Read the model definition and answer for the solid it produces. Units are mm, in the model's axes. Coordinates: 2 decimals unless noted, no trailing zeros. Loops run counter-clockwise (first coordinate to the right, second up) from the corner with the lowest first, then second, coordinate; pieces in that order, holes last. Notation, with made-up numbers: (61.25, -36) - (70.25, -36) arc R28 cw to (70.25, -15) - close; hole circle Ø8 at (-37.75, 28.25). An arc over 180 degrees is marked (long way). Use one line per item in the form item = value. Start each with the question number.
1) Each of these flat-tipped pins is pushed along its axis until it touches: P1, Ø3.5, axis at x = 137, y = 64, coming from the +Z side; P2, Ø1, axis at x = 16, z = 1.5, coming from the -Y side; P3, Ø1.5, axis at y = 72, z = 2, coming from the -X side. Where does it stop, or does it pass through?
2) A cutting plane is placed at A-A (y = 15). Give the vertices of the cut face in (x, z), and give its area (3 significant figures).
3) A cutting plane is placed at D-D (z = 2.1). State how many separate pieces and enclosed holes the cut face has, and give its area (3 significant figures).
4) The mould has two halves that part along X. Classify faces 1 (the face through (63, 37, 0)), 2 (the face through (106.05, 39.72, 1.52)), 3 (the face through (135.526, 65.352, 1.521)): released by +X, released by -X, zero draft, split by the parting line, or undercut.
5) Consider line 1 (X direction, y = 47.5, z = 1.45); line 2 (X direction, y = 66.5, z = 0.75); line 3 (Y direction, x = 88.5, z = 1.35). Determine where each line is inside the solid, lowest interval first.
6) A cutting plane is placed at C-C (y = 54). Give the vertices of the cut face in (x, z).
7) A cutting plane is placed at B-B (x = 137). Give the vertices of the cut face in (y, z).
from build123d import *

# Parameters (mm, degrees)
SKETCH1_R           = 5
BOSS_EXTRUDE1_DEPTH = 3
SKETCH2_R           = 2
SKETCH2_R_2         = 19
SKETCH2_W           = 4
SKETCH2_H           = 3
CUT_EXTRUDE1_DEPTH  = 10


with BuildPart() as part:
    # Sketch1 → Boss-Extrude1 (new body)
    with BuildSketch(Plane.XY):
        Polygon((30, 70), (0, 70), (-10, 70), (-10, 46.8), (-6.473616306, 46.8), (-6.473616306, 20.6), (-10, 20.6), (-10, 3), (0, 3), (30, 3), (30, 0), (60, 0), (60, 3), (90, 3), (90, 0), (120, 0), (120, 3), (150, 3), (150, 0), (180, 0), (180, 20.6), (177, 20.6), (177, 46.8), (180, 46.8), (180, 73), (150, 73), (150, 70), (120, 70), (120, 73), (90, 73), (90, 70), (60, 70), (60, 73), (30, 73), align=None)
        with Locations((145, 15)):
            Circle(SKETCH1_R, mode=Mode.SUBTRACT)
    extrude(amount=BOSS_EXTRUDE1_DEPTH)

    # Sketch2 → Cut-Extrude1 (cut)
    with BuildSketch(Plane.XY.offset(3)):
        with Locations((105.5, 64)):
            Circle(SKETCH2_R)
        with Locations((154, 47)):
            Circle(SKETCH2_R_2)
        with Locations((88.5, 47)):
            Circle(SKETCH2_R_2)
        with Locations((142, 68.5)):
            Rectangle(SKETCH2_W, SKETCH2_H)
        with BuildLine():
            Line((144, 67), (140, 67))
            Line((140, 67), (140, 65.5))
            ThreePointArc((140, 65.5), (142, 63.5), (144, 65.5))
            Line((144, 65.5), (144, 67))
        make_face()
        with Locations((71.5, 64)):
            Circle(SKETCH2_R)
        with Locations((71.5, 30)):
            Circle(SKETCH2_R)
        with Locations((105.5, 30)):
            Circle(SKETCH2_R)
        with Locations((137, 30)):
            Circle(SKETCH2_R)
        with Locations((171, 30)):
            Circle(SKETCH2_R)
        with Locations((171, 64)):
            Circle(SKETCH2_R)
        with Locations((137, 64)):
            Circle(SKETCH2_R)
        with BuildLine():
            Line((74.5, 70), (78.5, 70))
            Line((78.5, 70), (78.5, 65.5))
            ThreePointArc((78.5, 65.5), (76.5, 63.5), (74.5, 65.5))
            Line((74.5, 65.5), (74.5, 70))
        make_face()
    extrude(amount=-CUT_EXTRUDE1_DEPTH, mode=Mode.SUBTRACT)


solid = part.part
Found:
q1.P1 = through
q1.P2 = 3
q1.P3 = 30
q2.outline = (-10, 0) - (140, 0) - (140, 3) - (-10, 3) - close; (150, 0) - (180, 0) - (180, 3) - (150, 3) - close
q2.area = 540 mm^2
q3.separate_pieces = 1
q3.enclosed_holes = 11
q3.area = 10,600 mm^2
q4.face_1 = zero draft
q4.face_2 = undercut
q4.face_3 = undercut
q5.line_1 = -10 to 69.51, 107.49 to 135.01, 172.99 to 180
q5.line_2 = -10 to 74.5, 78.5 to 140, 144 to 180
q5.line_3 = 3 to 28, 66 to 70
q6.outline = (-10, 0) - (70.84, 0) - (70.84, 3) - (-10, 3) - close; (106.16, 0) - (136.34, 0) - (136.34, 3) - (106.16, 3) - close; (171.66, 0) - (180, 0) - (180, 3) - (171.66, 3) - close
q7.outline = (3, 0) - (28, 0) - (28, 3) - (3, 3) - close; (32, 0) - (38.51, 0) - (38.51, 3) - (32, 3) - close; (55.49, 0) - (62, 0) - (62, 3) - (55.49, 3) - close; (66, 0) - (70, 0) - (70, 3) - (66, 3) - close
